```python
from build123d import *

# Parameters (mm, degrees)
SKETCH1_W           = 6.35
SKETCH1_H           = 31.75
BOSS_EXTRUDE1_DEPTH = 50.8
BASE_MOUNTS_REACH   = 8.35
SKETCH2_R           = 3.96875
PEDAL_HINGE_REACH   = 8.35
SKETCH3_R           = 6.3627


with BuildPart() as part:
    # Sketch1 → Boss-Extrude1 (new body)
    with BuildSketch(Plane(origin=(0, 0, 0), x_dir=(0, 0, -1), z_dir=(1, 0, 0))):
        Polygon((6.35, 6.35), (6.35, 0), (38.1, 0), (38.1, 6.35), (31.75, 6.35), align=None)
        with Locations((34.925, 22.225)):
            Rectangle(SKETCH1_W, SKETCH1_H)
    extrude(amount=BOSS_EXTRUDE1_DEPTH)

    # Sketch2 → Base Mounts (cut, up to next)
    with BuildSketch(Plane(origin=(0, 6.35, 0), x_dir=(1, 0, 0), z_dir=(0, 1, 0)), mode=Mode.PRIVATE) as base_mounts_sk1:
        with Locations((38.1, 19.05)):
            Circle(SKETCH2_R)
    base_mounts_tool1 = extrude(base_mounts_sk1.sketch, amount=-BASE_MOUNTS_REACH, mode=Mode.PRIVATE) & part.part
    add(base_mounts_tool1.solids().sort_by_distance((38.1, 6.35, -19.05))[0], mode=Mode.SUBTRACT)
    # Sketch2 → Base Mounts (cut, up to next)
    with BuildSketch(Plane(origin=(0, 6.35, 0), x_dir=(1, 0, 0), z_dir=(0, 1, 0)), mode=Mode.PRIVATE) as base_mounts_sk2:
        with Locations((12.7, 19.05)):
            Circle(SKETCH2_R)
    base_mounts_tool2 = extrude(base_mounts_sk2.sketch, amount=-BASE_MOUNTS_REACH, mode=Mode.PRIVATE) & part.part
    add(base_mounts_tool2.solids().sort_by_distance((12.7, 6.35, -19.05))[0], mode=Mode.SUBTRACT)

    # Sketch3 → Pedal Hinge (cut, up to next)
    with BuildSketch(Plane.XY.offset(-31.75), mode=Mode.PRIVATE) as pedal_hinge_sk1:
        with Locations((25.4, 25.4)):
            Circle(SKETCH3_R)
    pedal_hinge_tool1 = extrude(pedal_hinge_sk1.sketch, amount=-PEDAL_HINGE_REACH, mode=Mode.PRIVATE) & part.part
    add(pedal_hinge_tool1.solids().sort_by_distance((25.4, 25.4, -31.75))[0], mode=Mode.SUBTRACT)
    # Sketch3 → Pedal Hinge (cut, up to next)
    with BuildSketch(Plane.XY.offset(-31.75), mode=Mode.PRIVATE) as pedal_hinge_sk2:
        Polygon((50.8, 6.35), (50.8, 38.1), (38.1, 38.1), align=None)
    pedal_hinge_tool2 = extrude(pedal_hinge_sk2.sketch, amount=-PEDAL_HINGE_REACH, mode=Mode.PRIVATE) & part.part
    add(pedal_hinge_tool2.solids().sort_by_distance((46.566667, 27.516667, -31.75))[0], mode=Mode.SUBTRACT)
    # Sketch3 → Pedal Hinge (cut, up to next)
    with BuildSketch(Plane.XY.offset(-31.75), mode=Mode.PRIVATE) as pedal_hinge_sk3:
        Polygon((0, 6.35), (0, 38.1), (12.7, 38.1), align=None)
    pedal_hinge_tool3 = extrude(pedal_hinge_sk3.sketch, amount=-PEDAL_HINGE_REACH, mode=Mode.PRIVATE) & part.part
    add(pedal_hinge_tool3.solids().sort_by_distance((4.233333, 27.516667, -31.75))[0], mode=Mode.SUBTRACT)


solid = part.part
```
Model file for the job. Use its own axes, mm. A direction names the side the tool comes from. Give positions to 0.01 mm unless a question says otherwise; leave off trailing zeros. Loops run counter-clockwise (first coordinate to the right, second up) from the corner with the lowest first, then second, coordinate; pieces in that order, holes last. Notation, with made-up numbers: (57, 85.5) -> (64, 85.5) arc R12 cw to (64, 103.5) -> close; hole circle Ø8 at (-29, 13). An arc over 180 degrees is marked (long way). Write each question's results on one line, items separated by ' | '.
(1) Flat gauge pins, fed straight in: pin 1 Ø9.5 at (x, y) = (26, 19.5) entering from +Z; pin 2 Ø8 at (y, z) = (5.5, -18) entering from -X; pin 3 Ø7.5 at (x, z) = (15.5, -25) entering from +Y. Where does each tip first touch, or does it go through?
Geometry results:
pin 1: stops at z = -31.75 | pin 2: stops at x = 0 | pin 3: stops at y = 6.35
(2) Cut at A-A on x = 25.4. List the corners of the cut face in (y, z), and give its area (3 significant figures).
Geometry results:
outline: (0, -38.1) -> (19.04, -38.1) -> (19.04, -31.75) -> (6.35, -31.75) -> (6.35, -6.35) -> (0, -6.35) -> close; (31.76, -38.1) -> (38.1, -38.1) -> (38.1, -31.75) -> (31.76, -31.75) -> close | area: 322 mm²
(3) Probe line 1 along X through (y, z) = (2, -19.05); line 2 along Z through (x, y) = (38.1, 1.5); line 3 along Y through (x, z) = (25.4, -34.75). List the from-to ranges inside material, lowest first.
Geometry results:
line 1: x = 0 to 8.73, 16.67 to 34.13, 42.07 to 50.8 | line 2: z = -38.1 to -23.02, -15.08 to -6.35 | line 3: y = 0 to 19.04, 31.76 to 38.1
(4) Cut at B-B on y = 25.4. List the corners of the cut face in (x, z), and give its area (3 significant figures).
Geometry results:
outline: (7.62, -38.1) -> (19.04, -38.1) -> (19.04, -31.75) -> (7.62, -31.75) -> close; (31.76, -38.1) -> (43.18, -38.1) -> (43.18, -31.75) -> (31.76, -31.75) -> close | area: 145 mm²
(5) Tool access for faces 1 (the flat face through (25, 6.35, -19)), 2 (the flat face through (44.36, 22.45, -34.88)): list every direction of +Z, -Z, +X, -X, +Y, -Y with a clear straight run to the whole face (end or side of a thin tool).
Geometry results:
face 1: +Z, +X, -X, +Y | face 2: +Z, -Z, +X, +Y
(6) Cut at C-C on z = -19.05. List the corners of the cut face in (x, y), and give its area (3 significant figures).
Geometry results:
outline: (0, 0) -> (8.73, 0) -> (8.73, 6.35) -> (0, 6.35) -> close; (16.67, 0) -> (34.13, 0) -> (34.13, 6.35) -> (16.67, 6.35) -> close; (42.07, 0) -> (50.8, 0) -> (50.8, 6.35) -> (42.07, 6.35) -> close | area: 222 mm²
(7) Pull direction Z, two halves, no side cores. Call faces 3 (the flat face through (6.44, 22.45, -34.88)), 4 (the flat face through (25, 15, -38.1)), 5 (the cylindrical face through (35.175, 3.219, -21.732)): released by +Z, released by -Z, zero draft, split by the parting line, or undercut.
Geometry results:
face 3: zero draft | face 4: released by -Z | face 5: undercut
(8) Cut at D-D on y = 5.5. List the corners of the cut face in (x, z).
Geometry results:
outline: (0, -38.1) -> (50.8, -38.1) -> (50.8, -6.35) -> (0, -6.35) -> close; hole circle Ø7.94 at (12.7, -19.05); hole circle Ø7.94 at (38.1, -19.05)
